```python
from build123d import *

# Parameters (mm, degrees)
ESQUISSE1_W             = 10.0584
ESQUISSE1_H             = 10.0584
BOSS_EXTRU_1_DEPTH      = 2.413
ESQUISSE2_W             = 5.334
ESQUISSE2_H             = 4.4196
ENL_V_MAT_EXTRU_1_DEPTH = 8.510544207
ESQUISSE3_W             = 1.143
ESQUISSE3_H             = 2.1336
ENL_V_MAT_EXTRU_2_DEPTH = 10.941918215
ESQUISSE4_W             = 1.0668
ESQUISSE4_H             = 1.8034
ENL_V_MAT_EXTRU_3_DEPTH = 1.143
ENL_V_MAT_EXTRU_4_DEPTH = 1.143
ESQUISSE6_W             = 1.0668
ESQUISSE6_H             = 4.4196
ENL_V_MAT_EXTRU_5_DEPTH = 8.510544207
ESQUISSE7_W             = 1.143
ESQUISSE7_H             = 2.1336
ENL_V_MAT_EXTRU_6_DEPTH = 10.078608125
PER_AGE1_D              = 1.1049
PER_AGE1_DEPTH          = 0.999998
PER_AGE2_D              = 1.1049
PER_AGE2_DEPTH          = 0.999998
PER_AGE3_D              = 1.1049
PER_AGE3_DEPTH          = 0.999998
ESQUISSE22_W            = 0.55245
ESQUISSE22_H            = 0.999998
PER_AGE5_D              = 1.1049
PER_AGE5_DEPTH          = 0.999998
PER_AGE6_D              = 1.1049
PER_AGE6_DEPTH          = 0.999998
PER_AGE7_D              = 1.1049
PER_AGE7_DEPTH          = 0.999998
PER_AGE8_D              = 1.1049
PER_AGE8_DEPTH          = 0.999998
CHANFREIN1_SIZE         = 0.20955
CHANFREIN1_SIZE2        = 0.362951247
CHANFREIN2_SIZE         = 0.20955
CHANFREIN2_SIZE2        = 0.362951247
CHANFREIN3_SIZE         = 0.20955
CHANFREIN3_SIZE2        = 0.362951247
CHANFREIN4_SIZE         = 0.20955
CHANFREIN4_SIZE2        = 0.362951247
CHANFREIN5_SIZE         = 0.20955
CHANFREIN5_SIZE_2       = 0.362951247
CHANFREIN6_SIZE         = 0.20955
CHANFREIN6_SIZE2        = 0.362951247
CHANFREIN7_SIZE         = 0.20955
CHANFREIN7_SIZE_2       = 0.362951247
CONG_1_R                = 0.762
CONG_2_R                = 0.762
CONG_3_R                = 0.762
CONG_4_R                = 0.762
CONG_5_R                = 0.762
CONG_6_R                = 0.762
CONG_7_R                = 0.762


with BuildPart() as part:
    # Esquisse1 → Boss.-Extru.1 (new body)
    with BuildSketch(Plane.XY):
        Rectangle(ESQUISSE1_W, ESQUISSE1_H)
    extrude(amount=-BOSS_EXTRU_1_DEPTH)

    # Esquisse2 → Enlèv. mat.-Extru.1 (cut, through all)
    with BuildSketch(Plane(origin=(0, 0, -2.413), x_dir=(-1, 0, 0), z_dir=(0, 0, -1))):
        with Locations((-0.5334, 0)):
            Rectangle(ESQUISSE2_W, ESQUISSE2_H)
    extrude(amount=-ENL_V_MAT_EXTRU_1_DEPTH, mode=Mode.SUBTRACT)

    # Esquisse3 → Enlèv. mat.-Extru.2 (cut, through all)
    with BuildSketch(Plane.ZY.offset(-3.2004)):
        with Locations((-0.5715, -0.6604)):
            Rectangle(ESQUISSE3_W, ESQUISSE3_H)
    extrude(amount=-ENL_V_MAT_EXTRU_2_DEPTH, mode=Mode.SUBTRACT)

    # Esquisse4 → Enlèv. mat.-Extru.3 (cut)
    with BuildSketch(Plane.XY):
        with Locations((4.4958, 1.3081)):
            Rectangle(ESQUISSE4_W, ESQUISSE4_H)
    extrude(amount=-ENL_V_MAT_EXTRU_3_DEPTH, mode=Mode.SUBTRACT)

    # Esquisse5 → Enlèv. mat.-Extru.4 (cut)
    with BuildSketch(Plane.XY):
        with BuildLine():
            Line((5.0292, -1.7272), (4.015471485, -1.7272))
            ThreePointArc((4.015471485, -1.7272), (4.295598647, -2.077699516), (4.7244, -2.2098))
            Line((4.7244, -2.2098), (5.0292, -2.2098))
            Line((5.0292, -2.2098), (5.0292, -1.7272))
        make_face()
    extrude(amount=-ENL_V_MAT_EXTRU_4_DEPTH, mode=Mode.SUBTRACT)

    # Esquisse6 → Enlèv. mat.-Extru.5 (cut, through all)
    with BuildSketch(Plane(origin=(0, 0, -2.413), x_dir=(-1, 0, 0), z_dir=(0, 0, -1))):
        with Locations((4.4958, 0)):
            Rectangle(ESQUISSE6_W, ESQUISSE6_H)
    extrude(amount=-ENL_V_MAT_EXTRU_5_DEPTH, mode=Mode.SUBTRACT)

    # Esquisse7 → Enlèv. mat.-Extru.6 (cut, through all)
    with BuildSketch(Plane(origin=(-2.1336, 0, 0), x_dir=(0, 0, -1), z_dir=(1, 0, 0))):
        with Locations((0.5715, -0.6604)):
            Rectangle(ESQUISSE7_W, ESQUISSE7_H)
    extrude(amount=-ENL_V_MAT_EXTRU_6_DEPTH, mode=Mode.SUBTRACT)

    # Esquisse8 → Révolution1 (revolve)
    with BuildSketch(Plane(origin=(0, -3.81, 0), x_dir=(-1, 0, 0), z_dir=(0, 1, 0))):
        Polygon((-4.064, -8.763), (-3.81, -8.763), (-3.81, -2.413), (-4.49834, -2.413), (-4.49834, -4.064), (-4.064, -4.318), align=None)
    revolve(axis=Axis((3.81, -3.81, -8.763), (0, 0, 1)))

    # Esquisse9 → Révolution2 (revolve)
    with BuildSketch(Plane(origin=(0, -3.81, 0), x_dir=(-1, 0, 0), z_dir=(0, 1, 0))):
        Polygon((-1.524, -7.366), (-1.27, -7.366), (-1.27, -2.413), (-1.95834, -2.413), (-1.95834, -4.064), (-1.524, -4.318), align=None)
    revolve(axis=Axis((1.27, -3.81, -7.366), (0, 0, 1)))

    # Esquisse10 → Révolution3 (revolve)
    with BuildSketch(Plane(origin=(0, -3.81, 0), x_dir=(-1, 0, 0), z_dir=(0, 1, 0))):
        Polygon((1.016, -8.763), (1.27, -8.763), (1.27, -2.413), (0.58166, -2.413), (0.58166, -4.064), (1.016, -4.318), align=None)
    revolve(axis=Axis((-1.27, -3.81, -8.763), (0, 0, 1)))

    # Esquisse11 → Révolution4 (revolve)
    with BuildSketch(Plane(origin=(0, -3.81, 0), x_dir=(-1, 0, 0), z_dir=(0, 1, 0))):
        Polygon((3.556, -8.763), (3.81, -8.763), (3.81, -2.413), (3.12166, -2.413), (3.12166, -4.064), (3.556, -4.318), align=None)
    revolve(axis=Axis((-3.81, -3.81, -8.763), (0, 0, 1)))

    # Esquisse12 → Révolution5 (revolve)
    with BuildSketch(Plane(origin=(0, 3.81, 0), x_dir=(-1, 0, 0), z_dir=(0, 1, 0))):
        Polygon((-4.064, -8.763), (-3.81, -8.763), (-3.81, -2.413), (-4.49834, -2.413), (-4.49834, -4.064), (-4.064, -4.318), align=None)
    revolve(axis=Axis((3.81, 3.81, -8.763), (0, 0, 1)))

    # Esquisse13 → Révolution6 (revolve)
    with BuildSketch(Plane(origin=(0, 3.81, 0), x_dir=(-1, 0, 0), z_dir=(0, 1, 0))):
        Polygon((-1.524, -8.763), (-1.27, -8.763), (-1.27, -2.413), (-1.95834, -2.413), (-1.95834, -4.064), (-1.524, -4.318), align=None)
    revolve(axis=Axis((1.27, 3.81, -8.763), (0, 0, 1)))

    # Esquisse14 → Révolution7 (revolve)
    with BuildSketch(Plane(origin=(0, 3.81, 0), x_dir=(-1, 0, 0), z_dir=(0, 1, 0))):
        Polygon((1.016, -7.366), (1.27, -7.366), (1.27, -2.413), (0.58166, -2.413), (0.58166, -4.064), (1.016, -4.318), align=None)
    revolve(axis=Axis((-1.27, 3.81, -7.366), (0, 0, 1)))

    # Esquisse15 → Révolution8 (revolve)
    with BuildSketch(Plane(origin=(0, 3.81, 0), x_dir=(-1, 0, 0), z_dir=(0, 1, 0))):
        Polygon((3.556, -8.763), (3.81, -8.763), (3.81, -2.413), (3.12166, -2.413), (3.12166, -4.064), (3.556, -4.318), align=None)
    revolve(axis=Axis((-3.81, 3.81, -8.763), (0, 0, 1)))

    # Perçage1
    with Locations(Plane.XY):
        with Locations((3.81, -3.81)):
            Hole(PER_AGE1_D / 2, depth=PER_AGE1_DEPTH)

    # Perçage2
    with Locations(Plane.XY):
        with Locations((-3.81, 3.81)):
            Hole(PER_AGE2_D / 2, depth=PER_AGE2_DEPTH)

    # Perçage3
    with Locations(Plane.XY):
        with Locations((1.27, -3.81)):
            Hole(PER_AGE3_D / 2, depth=PER_AGE3_DEPTH)

    # Esquisse22 → Perçage4 (revolve, cut)
    with BuildSketch(Plane(origin=(0, 3.81, 0), x_dir=(0, 0, 1), z_dir=(1, 0, 0))):
        with Locations((0.276225, 0.499999)):
            Rectangle(ESQUISSE22_W, ESQUISSE22_H)
    revolve(axis=Axis((0, -106.19, 0), (0, 1, 0)), mode=Mode.SUBTRACT)

    # Perçage5
    with Locations(Plane.XY):
        with Locations((-3.81, -3.81)):
            Hole(PER_AGE5_D / 2, depth=PER_AGE5_DEPTH)

    # Perçage6
    with Locations(Plane.XY):
        with Locations((1.27, 3.81)):
            Hole(PER_AGE6_D / 2, depth=PER_AGE6_DEPTH)

    # Perçage7
    with Locations(Plane.XY):
        with Locations((3.81, 3.81)):
            Hole(PER_AGE7_D / 2, depth=PER_AGE7_DEPTH)

    # Perçage8
    with Locations(Plane.XY):
        with Locations((-1.27, 3.81)):
            Hole(PER_AGE8_D / 2, depth=PER_AGE8_DEPTH)

    # Chanfrein1
    chanfrein1_edges = [part.edges().sort_by_distance(p)[0] for p in [
        (4.36245, -3.81, 0),
    ]]
    chanfrein1_side = [part.faces().sort_by_distance(p)[0] for p in [
        (-0.07802689, -3.515242334, 0),
    ]]
    chamfer(chanfrein1_edges, length=CHANFREIN1_SIZE, length2=CHANFREIN1_SIZE2, reference=chanfrein1_side[0])

    # Chanfrein2
    chanfrein2_edges = [part.edges().sort_by_distance(p)[0] for p in [
        (-3.25755, 3.81, 0),
    ]]
    chanfrein2_side = [part.faces().sort_by_distance(p)[0] for p in [
        (4.4958, 2.32049855, 0),
    ]]
    chamfer(chanfrein2_edges, length=CHANFREIN2_SIZE, length2=CHANFREIN2_SIZE2, reference=chanfrein2_side[0])

    # Chanfrein3
    chanfrein3_edges = [part.edges().sort_by_distance(p)[0] for p in [
        (1.82245, -3.81, 0),
    ]]
    chanfrein3_side = [part.faces().sort_by_distance(p)[0] for p in [
        (-0.207492952, -3.505427301, 0),
    ]]
    chamfer(chanfrein3_edges, length=CHANFREIN3_SIZE, length2=CHANFREIN3_SIZE2, reference=chanfrein3_side[0])

    # Chanfrein4
    chanfrein4_edges = [part.edges().sort_by_distance(p)[0] for p in [
        (-3.25755, -3.81, 0),
    ]]
    chanfrein4_side = [part.faces().sort_by_distance(p)[0] for p in [
        (-0.258386154, -3.494936097, 0),
    ]]
    chamfer(chanfrein4_edges, length=CHANFREIN4_SIZE, length2=CHANFREIN4_SIZE2, reference=chanfrein4_side[0])

    # Chanfrein5
    # the kernel refuses this chamfer: 0.362951247, 0.20955 mm, written as the material it takes off along each edge
    with BuildSketch(Plane(origin=(1.27, 3.81, 0), x_dir=(-1, 0, 0), z_dir=(0, -1, 0))) as chanfrein5_piece_1:
        Polygon((0.55245 + CHANFREIN5_SIZE, 0), (0.55245, CHANFREIN5_SIZE_2), (0.55245, 0), align=None)
    revolve(axis=Axis((1.27, 3.81, 0), (0, 0, -1)), mode=Mode.SUBTRACT)

    # Chanfrein6
    chanfrein6_edges = [part.edges().sort_by_distance(p)[0] for p in [
        (4.36245, 3.81, 0),
    ]]
    chanfrein6_side = [part.faces().sort_by_distance(p)[0] for p in [
        (4.4958, 2.32049855, 0),
    ]]
    chamfer(chanfrein6_edges, length=CHANFREIN6_SIZE, length2=CHANFREIN6_SIZE2, reference=chanfrein6_side[0])

    # Chanfrein7
    # the kernel refuses this chamfer: 0.362951247, 0.20955 mm, written as the material it takes off along each edge
    with BuildSketch(Plane(origin=(-1.27, 3.81, 0), x_dir=(-1, 0, 0), z_dir=(0, -1, 0))) as chanfrein7_piece_1:
        Polygon((0.55245 + CHANFREIN7_SIZE, 0), (0.55245, CHANFREIN7_SIZE_2), (0.55245, 0), align=None)
    revolve(axis=Axis((-1.27, 3.81, 0), (0, 0, -1)), mode=Mode.SUBTRACT)

    # Congé1
    cong_1_edges = [part.edges().sort_by_distance(p)[0] for p in [
        (-2.1336, -2.2098, -1.2065),
    ]]
    fillet(cong_1_edges, radius=CONG_1_R)

    # Congé2
    cong_2_edges = [part.edges().sort_by_distance(p)[0] for p in [
        (-3.9624, -2.2098, -1.2065),
    ]]
    fillet(cong_2_edges, radius=CONG_2_R)

    # Congé3
    cong_3_edges = [part.edges().sort_by_distance(p)[0] for p in [
        (-2.1336, 2.2098, -1.2065),
    ]]
    fillet(cong_3_edges, radius=CONG_3_R)

    # Congé4
    cong_4_edges = [part.edges().sort_by_distance(p)[0] for p in [
        (-3.9624, 2.2098, -1.2065),
    ]]
    fillet(cong_4_edges, radius=CONG_4_R)

    # Congé5
    cong_5_edges = [part.edges().sort_by_distance(p)[0] for p in [
        (3.2004, -2.2098, -1.2065),
    ]]
    fillet(cong_5_edges, radius=CONG_5_R)

    # Congé6
    cong_6_edges = [part.edges().sort_by_distance(p)[0] for p in [
        (3.9624, 2.2098, -0.5715),
    ]]
    fillet(cong_6_edges, radius=CONG_6_R)

    # Congé7
    cong_7_edges = [part.edges().sort_by_distance(p)[0] for p in [
        (3.2004, 2.2098, -1.2065),
    ]]
    fillet(cong_7_edges, radius=CONG_7_R)


solid = part.part
```
Here's how the part is built. I have some questions about the finished solid (model axes, mm). A direction names the side the tool comes from. Give positions to 0.01 mm unless a question says otherwise; leave off trailing zeros. Write each loop counter-clockwise with the first axis right and the second up, starting at its lowest first coordinate (ties: lowest second). Pieces come first, ordered by that corner, then holes. Notation, with made-up numbers: (-16.5, -8.5) -> (7.5, -8.5) arc R14 cw to (7.5, 2.5) -> close; hole circle Ø1 at (17, -30.5). An arc over 180 degrees is marked (long way). Write each question's results on one line, items separated by ' | '.
Item 1: Suppose I cut it at D-D on z = -6.5. Write out the boundary of the cut face in (x, y), plus the area to 3 significant figures.
Output:
outline: circle Ø0.51 at (-3.81, -3.81); circle Ø0.51 at (-3.81, 3.81); circle Ø0.51 at (-1.27, -3.81); circle Ø0.51 at (-1.27, 3.81); circle Ø0.51 at (1.27, -3.81); circle Ø0.51 at (1.27, 3.81); circle Ø0.51 at (3.81, -3.81); circle Ø0.51 at (3.81, 3.81) | area: 1.62 mm^2
Item 2: Suppose I cut it at C-C on y = -0.25. Write out the boundary of the cut face in (x, z), plus the area to 3 significant figures.
Output:
outline: (-3.96, -2.41) -> (-2.13, -2.41) -> (-2.13, -1.14) -> (-3.96, -1.14) -> close; (3.2, -2.41) -> (5.03, -2.41) -> (5.03, -1.14) -> (3.2, -1.14) -> close | area: 4.65 mm^2
Item 3: On a 3-axis mill with a long thin cutter (end or side, diameter ignored), from which of +Z, -Z, +X, -X, +Y, -Y can I reach the whole of each face in a straight line? I mean faces 1 (the face through (4.467, 4.017, -3.25)), 2 (the face through (4, -4, -1)), 3 (the face through (-3, -1, -1.143)). Say none if no direction works.
Output:
face 1: -Z | face 2: +Z | face 3: +Z, +X, -X
Item 4: Suppose I cut it at B-B on x = 0. Write out the boundary of the cut face in (y, z).
Output:
outline: (-5.03, -2.41) -> (-2.21, -2.41) -> (-2.21, 0) -> (-5.03, 0) -> close; (2.21, -2.41) -> (5.03, -2.41) -> (5.03, 0) -> (3.81, 0) -> (3.81, -0.55) -> (2.81, -0.55) -> (2.81, 0) -> (2.21, 0) -> close
Item 5: If I drill on L1, parallel to Y at x = 1.27, z = -0.8; L2, parallel to Y at x = 1.25, z = -4.5; L3, parallel to Z at x = -3.25, y = -3.25, over which ranges is the centre line in solid material (lowest first)?
Output:
L1: y = -5.03 to -4.36, -3.26 to -2.21, 2.21 to 3.26, 4.36 to 5.03 | L2: y = -4.06 to -3.56, 3.56 to 4.06 | L3: z = -2.41 to 0
Item 6: Suppose I cut it at A-A on z = -2.25. Write out the boundary of the cut face in (x, y).
Output:
outline: (-5.03, -5.03) -> (5.03, -5.03) -> (5.03, 5.03) -> (-5.03, 5.03) -> (-5.03, 2.21) -> (-4.72, 2.21) arc R0.76 cw to (-3.96, 1.45) -> (-3.96, -1.45) arc R0.76 cw to (-4.72, -2.21) -> (-5.03, -2.21) -> close; hole (-2.13, -1.45) arc R0.76 ccw to (-1.37, -2.21) -> (2.44, -2.21) arc R0.76 ccw to (3.2, -1.45) -> (3.2, 1.45) arc R0.76 ccw to (2.44, 2.21) -> (-1.37, 2.21) arc R0.76 ccw to (-2.13, 1.45) -> close
Item 7: We'd pull the mould along X, two halves only. Please class faces 4 (the face through (-4, 4, -1)), 5 (the face through (4, 0, -1.143)), 6 (the face through (-5.029, -4, -1)): pulls with the +X half, pulls with the -X half, needs draft (parallel to the pull), parting line crosses it, or undercut.
Output:
face 4: undercut | face 5: needs draft | face 6: pulls with the -X half
Item 8: For pin 1 Ø0.6 at (x, y) = (-3.5, -1) entering from +Z; pin 2 Ø1.9 at (y, z) = (-0.5, -1.5) entering from -X; pin 3 Ø3 at (x, z) = (2, -4.5) entering from -Y, each with a flat end and sliding along its axis, tell me the tip position at first contact or that it passes through.
Output:
pin 1: stops at z = -1.14 | pin 2: stops at x = -3.96 | pin 3: stops at y = -4.5
